Input: part model. Units: mm. Frame: model coordinates. Coordinates: 2 decimals unless noted, no trailing zeros. Write each loop counter-clockwise with the first axis right and the second up, starting at its lowest first coordinate (ties: lowest second). Pieces come first, ordered by that corner, then holes. Notation, with made-up numbers: (55.25, -11) - (75.25, -11) arc R22 ccw to (75.25, 17) - close; hole circle Ø1 at (-15, 51.25). An arc over 180 degrees is marked (long way). Put each result on its own line as item: value. Start each with the question number.
1. Line query: line 1 (Z direction, x = -730, y = -4); line 2 (X direction, y = -6.75, z = -196.5); line 3 (X direction, y = -3.75, z = 39). Output: solid intervals per line, ascending.
2. Pin query (flat end, axial travel): pin 1 (4 mm diameter, centred on y = -4.5, z = -125.5, fed in from -X); pin 2 (1.5 mm diameter, centred on y = -4.5, z = 287, fed in from +X); pin 3 (4 mm diameter, centred on x = -712, y = -2, fed in from -Z). Return the tip coordinate at first contact, or that it passes through.
3. Cut plane B-B, the plane z = 291. Return loops of the section in (x, y).
from build123d import *

# Parameters (mm, degrees)
F1_DEPTH = 7.9375
F2_R     = 0.635


with BuildPart() as f1:
    # F0 (on Front) → F1 (new body)
    with BuildSketch(Plane.XZ):
        with BuildLine():
            Line((-653.682642, -248.07856), (-665.9499, -251.365562))
            Line((-665.9499, -251.365562), (665.9499, -251.365562))
            Line((665.9499, -251.365562), (653.682642, -248.07856))
            Line((653.682642, -248.07856), (740.557894, -244.285505))
            ThreePointArc((740.557894, -244.285505), (781.50316, -225.733446), (798.251554, -184.017921))
            Line((798.251554, -184.017921), (798.251554, 160.088868))
            ThreePointArc((798.251554, 160.088868), (781.50316, 201.804393), (740.557894, 220.356452))
            Line((740.557894, 220.356452), (673.071263, 223.302982))
            ThreePointArc((673.071263, 223.302982), (666.999757, 229.785462), (673.348246, 235.996938))
            Line((673.348246, 235.996938), (790.988303, 235.996938))
            ThreePointArc((790.988303, 235.996938), (795.830132, 238.238509), (797.253598, 243.380659))
            ThreePointArc((797.253598, 243.380659), (753.87662, 319.965956), (671.251554, 350.296938))
            Line((671.251554, 350.296938), (-671.251554, 350.296938))
            ThreePointArc((-671.251554, 350.296938), (-753.87662, 319.965956), (-797.253598, 243.380659))
            ThreePointArc((-797.253598, 243.380659), (-795.830132, 238.238509), (-790.988303, 235.996938))
            Line((-790.988303, 235.996938), (-673.348246, 235.996938))
            ThreePointArc((-673.348246, 235.996938), (-666.999757, 229.785462), (-673.071263, 223.302982))
            Line((-673.071263, 223.302982), (-740.557894, 220.356452))
            ThreePointArc((-740.557894, 220.356452), (-781.50316, 201.804393), (-798.251554, 160.088868))
            Line((-798.251554, 160.088868), (-798.251554, 129.634438))
            ThreePointArc((-798.251554, 129.634438), (-790.812067, 111.673926), (-772.851554, 104.234438))
            Line((-772.851554, 104.234438), (-673.348246, 104.234438))
            ThreePointArc((-673.348246, 104.234438), (-664.36799, 100.514694), (-660.648246, 91.534438))
            Line((-660.648246, 91.534438), (-660.648246, -110.078062))
            ThreePointArc((-660.648246, -110.078062), (-664.36799, -119.058318), (-673.348246, -122.778062))
            Line((-673.348246, -122.778062), (-772.851554, -122.778062))
            ThreePointArc((-772.851554, -122.778062), (-790.812067, -130.21755), (-798.251554, -148.178062))
            Line((-798.251554, -148.178062), (-798.251554, -184.017921))
            ThreePointArc((-798.251554, -184.017921), (-781.50316, -225.733446), (-740.557894, -244.285505))
            Line((-740.557894, -244.285505), (-653.682642, -248.07856))
        make_face()
    extrude(amount=F1_DEPTH)

    # F2
    f2_edges = [f1.edges().sort_by_distance(p)[0] for p in [
        (-653.682642, -3.96875, -248.07856),
        (653.682642, -3.96875, -248.07856),
    ]]
    fillet(f2_edges, radius=F2_R)


solid = f1.part
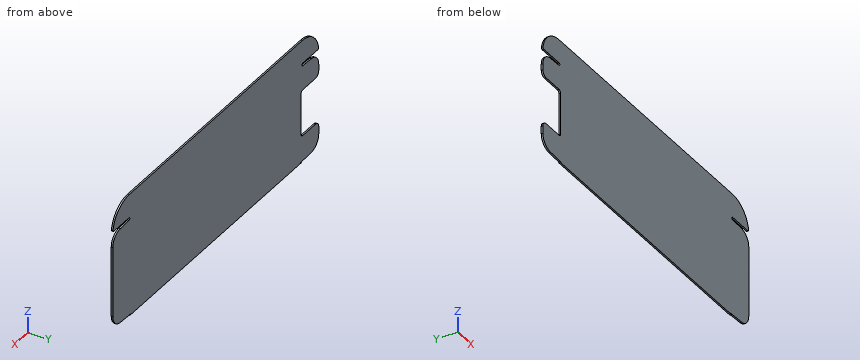
Report:
1. line 1: z = -244.75 to -122.78, 104.23 to 220.82, 236 to 335.98
1. line 2: x = -796.95 to 796.95
1. line 3: x = -660.65 to 798.25
2. pin 1: stops at x = -787.6
2. pin 2: stops at x = 781.96
2. pin 3: stops at z = -245.62
3. outline: (-779.09, -7.94) - (779.09, -7.94) - (779.09, 0) - (-779.09, 0) - close
